Autodesk Inventor part; units mm, degrees
ref_plane "YZ Plane" through (0, 0, 0) normal (1, 0, 0) x (0, 1, 0)
ref_plane "XZ Plane" through (0, 0, 0) normal (0, 1, 0) x (-1, 0, 0)
ref_plane "XY Plane" through (0, 0, 0) normal (0, 0, 1) x (1, 0, 0)
sketch "Szkic1" plane through (0, 0, 0) normal (0, 0, 1) x (1, 0, 0)
  circle A0 centre (0, 0) radius 27.5
  dimension "d0" = 55
extrude "Wyciągnięcie proste1" add sketch "Szkic1" along normal mid plane 10
sketch "Szkic3" plane through (0, 0, 0) normal (0, 0, 1) x (1, 0, 0)
  circle A0 centre (0, 0) radius 32.5
  circle A1 centre (0, 0) radius 27.5
  dimension "d4" = 65
  dimension "d5" = 55
extrude "Wyciągnięcie proste2" add sketch "Szkic3" along normal mid plane 15
sketch "Szkic4" plane through (0, 0, -7.5) normal (0, 0, -1) x (-1, 0, 0)
  point P0 (0, 0)
  point P1 (0, 0)
hole "Otwór1" at (0, 0, -7.5) direction (0, 0, 1) diameter 5 end through all
properties part number "Koło" material "Tworzywo sztuczne PET"
Verification items for the finished model (mm, model axes). A direction names the side the tool comes from. Give positions to 0.01 mm unless a question says otherwise; leave off trailing zeros. Write each loop counter-clockwise with the first axis right and the second up, starting at its lowest first coordinate (ties: lowest second). Pieces come first, ordered by that corner, then holes. Notation, with made-up numbers: M -33.75,36 L 18.25,36 A37 ccw 18.25,74 Z; hole C 84,38 d7. An arc over 180 degrees is marked long. Use CSV: the item, a comma, the result in double quotes.
1) Access from +Z, -Z, +X, -X, +Y, -Y to the whole of each face (thin tool, end or side, straight path). Record for faces 4 (the face through (-27, 7, 7.5)), 5 (the face through (-5.961, 26.846, 6.232)), 6 (the face through (-5.961, -26.846, -6.232)).
Final values:
face 4,"+Z, +X, -X, +Y, -Y"
face 5,"+Z"
face 6,"-Z"
2) Go/stop test with flat-tipped pins: pin 1 Ø1.5 at (x, z) = (4.5, -2.5) entering from -Y; pin 2 Ø6 at (y, z) = (-7.5, -1.5) entering from +X; pin 3 Ø6.5 at (x, y) = (0, 0) entering from -Z. Record where each tip stops, or that it passes through.
Final values:
pin 1,"y = -32.28"
pin 2,"x = 32.19"
pin 3,"z = -5"
3) Cross-section at A-A (y = 0). Enter the section's corners in (x, z).
Final values:
outline,"M -32.5,-7.5 L -27.5,-7.5 L -27.5,-5 L -2.5,-5 L -2.5,5 L -27.5,5 L -27.5,7.5 L -32.5,7.5 Z; M 2.5,-5 L 27.5,-5 L 27.5,-7.5 L 32.5,-7.5 L 32.5,7.5 L 27.5,7.5 L 27.5,5 L 2.5,5 Z"
4) Release check for a two-part mould opening along Y. For faces 1 (the face through (-27, 7, -7.5)), 2 (the face through (31, 9.76, 0.11)), 3 (the face through (0, -6, -5)) record: released by +Y, released by -Y, zero draft, split by the parting line, or undercut.
Final values:
face 1,"zero draft"
face 2,"split by the parting line"
face 3,"undercut"
5) Cross-section at C-C (x = 16.5). Enter the section's corners in (y, z).
Final values:
outline,"M -28,-7.5 L -22,-7.5 L -22,-5 L 22,-5 L 22,-7.5 L 28,-7.5 L 28,7.5 L 22,7.5 L 22,5 L -22,5 L -22,7.5 L -28,7.5 Z"
6) Cross-section at D-D (z = -6.5). Enter the section's corners in (x, y).
Final values:
outline,"C 0,0 d65; hole C 0,0 d55"
7) Material ranges on line 1 along Y through (x, z) = (0, 0.5); line 2 along Z through (x, y) = (12.5, -13.5); line 3 along X through (y, z) = (-13.5, 6.25), recorded low to high.
Final values:
line 1,"-32.5 to -2.5, 2.5 to 32.5"
line 2,"-5 to 5"
line 3,"-29.56 to -23.96, 23.96 to 29.56"
